Geometry check sheet. Reference: the model listing, model coordinates, mm. Face numbers are marked on the shaded views. A direction names the side the tool comes from. Round coordinates to 2 decimals unless told otherwise and drop trailing zeros. Loops run counter-clockwise (first coordinate to the right, second up) from the corner with the lowest first, then second, coordinate; pieces in that order, holes last. Notation, with made-up numbers: (-30.75, 64) -> (12.25, 64) arc R21 ccw to (12.25, 79) -> close; hole circle Ø4 at (-24, -7.5). An arc over 180 degrees is marked (long way). Use a Markdown table: item, result. Add a question column.
Q1. Sectioned sample at A-A, the plane x = 69.5. Enter the section's corners in (y, z), then the cut area to 3 significant figures.
Q2. Set-up check for the marked faces 1 and 2: record each of +Z, -Z, +X, -X, +Y, -Y from which the full face is reachable in a straight line by a thin tool's end or side.
Q3. Material ranges on L1, parallel to Z at x = -66.5, y = 26; L2, parallel to Z at x = -22.5, y = 7; L3, parallel to Z at x = -10, y = -4.5, recorded low to high.
Q4. Gauge pin test, flat ends, axial feed: P1, Ø18, axis at y = 1, z = 1, coming from the +X side; P2, Ø0.5, axis at x = -55.5, y = -6, coming from the +Z side; P3, Ø3, axis at x = 55, y = -32.5, coming from the +Z side. Record the tip position at first contact, or that the pin passes through.
Q5. Sectioned sample at B-B, the plane y = 36. Enter the section's corners in (x, z), then the cut area to 3 significant figures.
Q6. Release check for a two-part mould opening along Z. For the marked faces 3, 4 and 5 record: released by +Z, released by -Z, zero draft, split by the parting line, or undercut.
Q7. Sectioned sample at C-C, the plane z = -43. Enter the section's corners in (x, y), then the cut area to 3 significant figures.
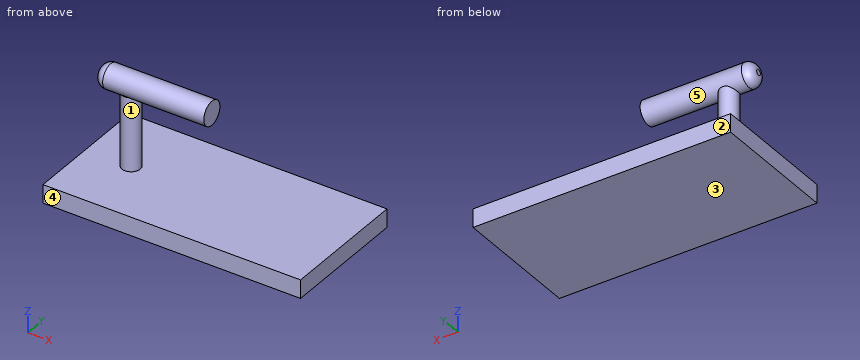
```python
from build123d import *

# Parameters (mm, degrees)
F0_W     = 177.8
F0_H     = 12.7
F1_DEPTH = 44.45
F2_R     = 6.35
F3_DEPTH = 50.8
F4_R     = 10.728509
F5_DEPTH = 127
F6_R     = 8.265321
F7_DEPTH = 76.2
F8_R     = 6.35


with BuildPart() as f1:
    # F0 (on Front) → F1 (new body, symmetric)
    with BuildSketch(Plane.XZ):
        with Locations((2.174042, -62.946092)):
            Rectangle(F0_W, F0_H)
    extrude(amount=F1_DEPTH, both=True)

    # F2 (on face) → F3 (join)
    with BuildSketch(Plane.XY.offset(-56.596092)):
        with Locations((-55.75341, 0)):
            Circle(F2_R)
    extrude(amount=F3_DEPTH)

    # F4 (on Right) → F5 (cut)
    with BuildSketch(Plane.YZ):
        with Locations((0, 3.137364)):
            Circle(F4_R)
    extrude(amount=-F5_DEPTH, mode=Mode.SUBTRACT)

    # F6 (on Right) → F7 (join)
    with BuildSketch(Plane.YZ):
        Circle(F6_R)
    extrude(amount=-F7_DEPTH)

    # F8
    f8_edges = [f1.edges().sort_by_distance(p)[0] for p in [
        (-76.2, -8.265321, 0),
    ]]
    fillet(f8_edges, radius=F8_R)


solid = f1.part
```
Values:
| question | item | result |
|---|---|---|
| 1 | outline | (-44.45, -69.3) -> (44.45, -69.3) -> (44.45, -56.6) -> (-44.45, -56.6) -> close |
| 1 | area | 1,130 mm^2 |
| 2 | face 1 | none |
| 2 | face 2 | +Z, -Z, +X, -X, +Y |
| 3 | L1 | -69.3 to -56.6 |
| 3 | L2 | -69.3 to -56.6, -4.39 to 4.39 |
| 3 | L3 | -69.3 to -56.6, -6.93 to 6.93 |
| 4 | P1 | x = 0 |
| 4 | P2 | z = 5.94 |
| 4 | P3 | z = -56.6 |
| 5 | outline | (-86.73, -69.3) -> (91.07, -69.3) -> (91.07, -56.6) -> (-86.73, -56.6) -> close |
| 5 | area | 2,260 mm^2 |
| 6 | face 3 | released by -Z |
| 6 | face 4 | zero draft |
| 6 | face 5 | undercut |
| 7 | outline | circle Ø12.7 at (-55.75, 0) |
| 7 | area | 127 mm^2 |
